Check sheet for the modelled part. Datum: model origin and axes. Units: mm. A direction names the side the tool comes from. Give positions to 0.01 mm unless a question says otherwise; leave off trailing zeros. Write each loop counter-clockwise with the first axis right and the second up, starting at its lowest first coordinate (ties: lowest second). Pieces come first, ordered by that corner, then holes. Notation, with made-up numbers: M 51.5,33 L 77.5,33 A21 cw 77.5,55 Z; hole C 26,37 d4. An arc over 180 degrees is marked long. Write item = value, one per line. Start each with the question number.
1) Sectioned sample at C-C, the plane x = 0. Record the cut outline in (y, z), then the cut area to 3 significant figures.
2) Gauge pin test, flat end, axial feed: pin 1 (2 mm diameter, centred on x = 7.77, y = -12.74, fed in from -Z). Record the tip position at first contact, or that the pin passes through.
3) Scan lines: L1, parallel to X at y = 1.5, z = -0.3; L2, parallel to Y at x = -11, z = 0.5; L3, parallel to X at y = 5, z = -0.6. Record each from-to range of solid material in increasing order.
4) Draft check along X on faces 1 (the face through (-0.687, 18.237, 0.01)), 2 (the face through (3, 15, -0.75)), 3 (the face through (-7.366, -16.432, -0.01)). Enter one of: pulls with the +X half, pulls with the -X half, needs draft (parallel to the pull), parting line crosses it, or undercut.
5) Sectioned sample at D-D, the plane y = 3. Record the cut outline in (x, z), then the cut area to 3 significant figures.
6) Set-up check for faces 4 (the face through (-11.48, -11.11, 0.01)), 5 (the face through (3, 15, 0.75)), 6 (the face through (6.4, -14.8, 0)): record each of +Z, -Z, +X, -X, +Y, -Y from which the full face is reachable in a straight line by a thin tool's end or side.
7) Sectioned sample at A-A, the plane y = 8. Record the cut outline in (x, z).
8) Sectioned sample at B-B, the plane z = -0.5. Count the separate pieces of the cut face and the enclosed holes in it, then the cut area to 3 significant figures.
from build123d import *

# Parameters (mm, degrees)
SKETCH3_R                = 1.25
BOSS_EXTRUDE1_DEPTH      = 0.75
BOSS_EXTRUDE1_DEPTH_BACK = 0.75
FILLET1_R                = 0.79375


with BuildPart() as part:
    # Sketch3 → Boss-Extrude1 (new body, two sides)
    with BuildSketch(Plane.XY) as boss_extrude1_sk:
        with BuildLine():
            Line((-5.8660137, -13.566130003), (-7.243190661, -16.751080235))
            ThreePointArc((-7.243190661, -16.751080235), (0, 18.25), (7.243190661, -16.751080235))
            Line((7.243190661, -16.751080235), (5.8660137, -13.566130003))
            ThreePointArc((5.8660137, -13.566130003), (6.338884196, -11.240641223), (8.684339918, -10.879612098))
            ThreePointArc((8.684339918, -10.879612098), (11.441621609, -11.12015326), (13.643394773, -9.443055377))
            ThreePointArc((13.643394773, -9.443055377), (0, 14.95), (-13.643394773, -9.443055377))
            ThreePointArc((-13.643394773, -9.443055377), (-11.441621609, -11.12015326), (-8.684339918, -10.879612098))
            ThreePointArc((-8.684339918, -10.879612098), (-6.338884196, -11.240641223), (-5.8660137, -13.566130003))
        make_face()
        with Locations((-7.770588576, -12.742589147)):
            Circle(SKETCH3_R, mode=Mode.SUBTRACT)
        with Locations((7.770588576, -12.742589147)):
            Circle(SKETCH3_R, mode=Mode.SUBTRACT)
    extrude(amount=BOSS_EXTRUDE1_DEPTH)
    extrude(boss_extrude1_sk.sketch, amount=-BOSS_EXTRUDE1_DEPTH_BACK)

    # Fillet1
    fillet1_edges = [part.edges().sort_by_distance(p)[0] for p in [
        (7.243190661, -16.751080235, 0),
        (-7.243190661, -16.751080235, 0),
    ]]
    fillet(fillet1_edges, radius=FILLET1_R)


solid = part.part
Data:
q1.outline = M 14.95,-0.75 L 18.25,-0.75 L 18.25,0.75 L 14.95,0.75 Z
q1.area = 4.95 mm2
q2.pin_1 = through
q3.L1 = -18.19 to -15.81, 15.81 to 18.19
q3.L2 = -14.56 to -11.22, 10.57 to 14.56
q3.L3 = -17.55 to -14.82, 14.82 to 17.55
q4.face_1 = parting line crosses it
q4.face_2 = needs draft
q4.face_3 = undercut
q5.outline = M -18,-0.75 L -15.49,-0.75 L -15.49,0.75 L -18,0.75 Z; M 15.49,-0.75 L 18,-0.75 L 18,0.75 L 15.49,0.75 Z
q5.area = 7.54 mm2
q6.face_4 = +Z, -Z
q6.face_5 = +Z, +X, -X, +Y, -Y
q6.face_6 = +Z, -Z, -Y
q7.outline = M -16.4,-0.75 L -13.2,-0.75 L -13.2,0.75 L -16.4,0.75 Z; M 13.2,-0.75 L 16.4,-0.75 L 16.4,0.75 L 13.2,0.75 Z
q8.separate_pieces = 1
q8.enclosed_holes = 2
q8.area = 251 mm2
